Design review of the part built by this model. Coordinates are the model's own, in mm. A direction names the side the tool comes from. Coordinates: 2 decimals unless noted, no trailing zeros. Write each loop counter-clockwise with the first axis right and the second up, starting at its lowest first coordinate (ties: lowest second). Pieces come first, ordered by that corner, then holes.
Q1. Add section D-D, the plane y = 45.5. Give the boundary of the cut face in (x, z), plus the area to 3 significant figures.
Q2. To check wall thickness, follow probe 1 along X at (y, z) = (-18, 26); probe 2 along Y at (x, z) = (90.5, 26.5); probe 3 along X at (y, z) = (-51, 7). State the ranges of each line that lie inside material, in increasing order.
Q3. Add section A-A, the plane x = -84.5. Give the boundary of the cut face in (y, z).
Q4. The part is to be moulded in two halves that separate along Y. For faces 5 (the face through (-2, -61, 15)), 6 (the face through (129.035, 46.584, 15.415)), 7 (the face through (-1, -58, 0)), 8 (the face through (-129, 31, 11)), say which applies: +Y half, -Y half, draft (parallel to the pull), parting line (faces both ways), or undercut.
Q5. Machinability: for faces 1 (the face through (-116, 1, 33.4)), 2 (the face through (124.5, -17, 15)), 3 (the face through (-43.35, 36.99, 31.68)), 4 (the face through (-128.965, -43.416, 15.415)), which of the approach directions +Z, -Z, +X, -X, +Y, -Y give a long, thin tool a straight path to every point of the face, cutting with its end or side? Answer none if there is none.
Q6. Add section C-C, the plane x = -10. Give the boundary of the cut face in (y, z), plus the area to 3 significant figures.
Q7. Clearance check with flat-ended pins moving along their axes: pin 1 Ø6.5 at (x, y) = (-3, 31.5) entering from -Z; pin 2 Ø1.2 at (x, z) = (-127, 5) entering from -Y; pin 3 Ø6 at (x, z) = (22, 30.5) entering from -Y; pin 4 Ø2 at (x, y) = (99.5, -31) entering from -Z. State where each tip first meets the part, or that it passes through.
Q8. Add section B-B, the plane y = 0. Give the number of separate pieces and of enclosed holes in the cut face, plus the area to 3 significant figures.
from build123d import *

# Parameters (mm, degrees)
SKETCH1_W             = 263
SKETCH1_H             = 122
SKETCH1_W_2           = 253
SKETCH1_H_2           = 112
BOSS_EXTRUDE1_DEPTH   = 30
SKETCH1_W_3           = 249
SKETCH1_H_3           = 108
SKETCH1_W_4           = 239
SKETCH1_H_4           = 98
BOSS_EXTRUDE1_2_DEPTH = 30
SKETCH2_W             = 263
SKETCH2_H             = 122
BOSS_EXTRUDE2_DEPTH   = 5
FILLET1_R             = 1.5
SKETCH3_R             = 17.5
CUT_EXTRUDE1_DEPTH    = 12
FILLET2_R             = 3.5
FILLET3_R             = 8.5
FILLET4_R             = 5
SKETCH4_R             = 2.35
CUT_EXTRUDE2_DEPTH    = 279
SKETCH5_W             = 20
SKETCH5_H             = 35
CUT_EXTRUDE3_DEPTH    = 30
SKETCH6_W             = 7.5
SKETCH6_H             = 9
SKETCH6_W_2           = 22.5
CUT_EXTRUDE4_DEPTH    = 2.5
SKETCH7_R             = 5
CUT_EXTRUDE8_DEPTH    = 73.5
SKETCH9_R             = 3
SKETCH9_R_2           = 1.25
BOSS_EXTRUDE4_DEPTH   = 4
SKETCH10_W            = 81
SKETCH10_H            = 53
CUT_EXTRUDE9_DEPTH    = 13.6
SKETCH11_W            = 90
SKETCH11_H            = 100
CUT_EXTRUDE10_DEPTH   = 1.6
SKETCH12_W            = 70
SKETCH12_H            = 80
CUT_EXTRUDE11_DEPTH   = 11.6
FILLET5_R             = 10


with BuildPart() as part:
    # Sketch1 → Boss-Extrude1 (new body)
    with BuildSketch(Plane.XY):
        Rectangle(SKETCH1_W, SKETCH1_H)
        Rectangle(SKETCH1_W_2, SKETCH1_H_2, mode=Mode.SUBTRACT)
    extrude(amount=BOSS_EXTRUDE1_DEPTH)



with BuildPart() as body_2:
    # Sketch1 → Boss-Extrude1 2 (new body)
    with BuildSketch(Plane.XY):
        Rectangle(SKETCH1_W_3, SKETCH1_H_3)
        Rectangle(SKETCH1_W_4, SKETCH1_H_4, mode=Mode.SUBTRACT)
    extrude(amount=BOSS_EXTRUDE1_2_DEPTH)


with BuildPart() as part_1:
    add(part.part)

    add(body_2.part)  # Boss-Extrude2 merges body 2
    # Sketch2 → Boss-Extrude2 (add)
    with BuildSketch(Plane.XY.offset(30)):
        Rectangle(SKETCH2_W, SKETCH2_H)
    extrude(amount=BOSS_EXTRUDE2_DEPTH)

    # Fillet1
    fillet1_edges = [part_1.edges().sort_by_distance(p)[0] for p in [
        (-124.5, -54, 15),
        (124.5, -54, 15),
        (124.5, 54, 15),
        (-124.5, 54, 15),
    ]]
    fillet(fillet1_edges, radius=FILLET1_R)

    # Sketch3 → Cut-Extrude1 (cut)
    with BuildSketch(Plane(origin=(0, -61, 0), x_dir=(-1, 0, 0), z_dir=(0, -1, 0))):
        with Locations((105, -7.5)):
            Circle(SKETCH3_R)
        with Locations((-105, -7.5)):
            Circle(SKETCH3_R)
    extrude(amount=-CUT_EXTRUDE1_DEPTH, mode=Mode.SUBTRACT)

    # Fillet2
    fillet2_edges = [part_1.edges().sort_by_distance(p)[0] for p in [
        (126.5, 56, 15),
        (-126.5, 56, 15),
        (-126.5, -56, 15),
        (126.5, -56, 15),
    ]]
    fillet(fillet2_edges, radius=FILLET2_R)

    # Fillet3
    fillet3_edges = [part_1.edges().sort_by_distance(p)[0] for p in [
        (-131.5, -61, 17.5),
        (-131.5, 61, 17.5),
        (131.5, 61, 17.5),
        (131.5, -61, 17.5),
    ]]
    fillet(fillet3_edges, radius=FILLET3_R)

    # Fillet4
    fillet4_edges = [part_1.edges().sort_by_distance(p)[0] for p in [
        (0, -61, 35),
        (-131.5, 0, 35),
        (131.5, 0, 35),
        (0, 61, 35),
        (-129.01040764, 58.51040764, 35),
        (129.01040764, 58.51040764, 35),
        (129.01040764, -58.51040764, 35),
        (-129.01040764, -58.51040764, 35),
    ]]
    fillet(fillet4_edges, radius=FILLET4_R)

    # Sketch4 → Cut-Extrude2 (cut)
    with BuildSketch(Plane(origin=(131.5, 0, 0), x_dir=(0, 0, -1), z_dir=(1, 0, 0))):
        with Locations(Location((-17.5, -44.5, 0), (0, 0, 90))):
            Circle(SKETCH4_R)
        with Locations(Location((-17.5, 45.5, 0), (0, 0, 90))):
            Circle(SKETCH4_R)
    extrude(amount=-CUT_EXTRUDE2_DEPTH, mode=Mode.SUBTRACT)

    # Sketch5 → Cut-Extrude3 (cut)
    with BuildSketch(Plane(origin=(0, 0, 0), x_dir=(-1, 0, 0), z_dir=(0, 0, -1))):
        with Locations((114.5, 36.5)):
            Rectangle(SKETCH5_W, SKETCH5_H)
        with Locations((-114.5, 36.5)):
            Rectangle(SKETCH5_W, SKETCH5_H)
    extrude(amount=-CUT_EXTRUDE3_DEPTH, mode=Mode.SUBTRACT)

    # Sketch6 → Cut-Extrude4 (cut)
    with BuildSketch(Plane(origin=(-126.5, 0, 0), x_dir=(0, 0, -1), z_dir=(1, 0, 0))):
        with Locations((-3.75, 45.5)):
            Rectangle(SKETCH6_W, SKETCH6_H)
        with Locations((-11.25, 30.5)):
            Rectangle(SKETCH6_W_2, SKETCH6_H)
    extrude(amount=-CUT_EXTRUDE4_DEPTH, mode=Mode.SUBTRACT)

    # Sketch7 → Cut-Extrude8 (cut)
    with BuildSketch(Plane.XY.offset(30)):
        with Locations(Location((104, 20, 0), (0, 0, 180))):
            Circle(SKETCH7_R)
        with Locations(Location((104, 0, 0), (0, 0, 180))):
            Circle(SKETCH7_R)
        with Locations(Location((104, -20, 0), (0, 0, 180))):
            Circle(SKETCH7_R)
    extrude(amount=CUT_EXTRUDE8_DEPTH, mode=Mode.SUBTRACT)

    # Sketch9 → Boss-Extrude4 (add)
    # profile 1 of 4: a face of its own
    with BuildSketch(Plane(origin=(0, 0, 30), x_dir=(-1, 0, 0), z_dir=(0, 0, -1))):
        with Locations((-84.5, 32)):
            Circle(SKETCH9_R)
        with Locations((-84.5, 32)):
            Circle(SKETCH9_R_2, mode=Mode.SUBTRACT)
    # profile 2 of 4: a face of its own
    with BuildSketch(Plane(origin=(0, 0, 30), x_dir=(-1, 0, 0), z_dir=(0, 0, -1))):
        with Locations((-84.5, -32)):
            Circle(SKETCH9_R)
        with Locations((-84.5, -32)):
            Circle(SKETCH9_R_2, mode=Mode.SUBTRACT)
    # profile 3 of 4: a face of its own
    with BuildSketch(Plane(origin=(0, 0, 30), x_dir=(-1, 0, 0), z_dir=(0, 0, -1))):
        with Locations((3.5, -32)):
            Circle(SKETCH9_R)
        with Locations((3.5, -32)):
            Circle(SKETCH9_R_2, mode=Mode.SUBTRACT)
    # profile 4 of 4: a face of its own
    with BuildSketch(Plane(origin=(0, 0, 30), x_dir=(-1, 0, 0), z_dir=(0, 0, -1))):
        with Locations((3.5, 32)):
            Circle(SKETCH9_R)
        with Locations((3.5, 32)):
            Circle(SKETCH9_R_2, mode=Mode.SUBTRACT)
    extrude(amount=BOSS_EXTRUDE4_DEPTH)

    # Sketch10 → Cut-Extrude9 (cut)
    with BuildSketch(Plane(origin=(0, 0, 30), x_dir=(-1, 0, 0), z_dir=(0, 0, -1))):
        with Locations((-40.5, 0)):
            Rectangle(SKETCH10_W, SKETCH10_H)
    extrude(amount=-CUT_EXTRUDE9_DEPTH, mode=Mode.SUBTRACT)

    # Sketch11 → Cut-Extrude10 (cut)
    with BuildSketch(Plane.XY.offset(35)):
        with Locations((-75.5, 0)):
            Rectangle(SKETCH11_W, SKETCH11_H)
    extrude(amount=-CUT_EXTRUDE10_DEPTH, mode=Mode.SUBTRACT)

    # Sketch12 → Cut-Extrude11 (cut)
    with BuildSketch(Plane.XY.offset(33.4)):
        with Locations((-75.5, 0)):
            Rectangle(SKETCH12_W, SKETCH12_H)
    extrude(amount=-CUT_EXTRUDE11_DEPTH, mode=Mode.SUBTRACT)

    # Fillet5
    fillet5_edges = [part_1.edges().sort_by_distance(p)[0] for p in [
        (-30.5, 50, 34.2),
        (-30.5, -50, 34.2),
        (-120.5, -50, 34.2),
        (-120.5, 50, 34.2),
        (-110.5, -40, 31.7),
        (-110.5, 40, 31.7),
        (-40.5, 40, 31.7),
        (-40.5, -40, 31.7),
    ]]
    fillet(fillet5_edges, radius=FILLET5_R)


solid = part_1.part
Here are the results:
1. outline: (-131.5, 0) - (-129, 0) - (-129, 7.5) - (-126.5, 7.5) - (-126.5, 15.15) - (-131.5, 15.15) - close; (-131.5, 19.85) - (-126.5, 19.85) - (-126.5, 30) - (126.5, 30) - (126.5, 19.85) - (131.5, 19.85) - (131.5, 30) arc R5 ccw to (126.5, 35) - (-32.15, 35) - (-32.15, 33.4) - (-118.85, 33.4) - (-118.85, 35) - (-126.5, 35) arc R5 ccw to (-131.5, 30) - close; (126.5, 0) - (131.5, 0) - (131.5, 15.15) - (126.5, 15.15) - close
1. area: 1,400 mm2
2. probe 1: x = -131.5 to -126.5, -124.5 to -119.5, 119.5 to 124.5, 126.5 to 131.5
2. probe 2: y = -61 to -56, -54 to -49, 49 to 54, 56 to 61
2. probe 3: x = -131.5 to -126.5, -124.5 to -122.49, -87.51 to 87.51, 122.49 to 124.5, 126.5 to 131.5
3. outline: (-61, 0) - (-56, 0) - (-56, 30) - (-54, 30) - (-54, 0) - (-49, 0) - (-49, 30) - (-40, 30) - (-40, 33.4) - (-50, 33.4) - (-50, 35) - (-56, 35) arc R5 ccw to (-61, 30) - close; (40, 30) - (49, 30) - (49, 0) - (54, 0) - (54, 30) - (56, 30) - (56, 0) - (61, 0) - (61, 30) arc R5 ccw to (56, 35) - (50, 35) - (50, 33.4) - (40, 33.4) - close
4. face 5: -Y half
4. face 6: undercut
4. face 7: draft
4. face 8: undercut
5. face 1: +Z
5. face 2: -Z
5. face 3: +Z, -Z
5. face 4: +X, -X
6. outline: (-61, 0) - (-56, 0) - (-56, 30) - (-54, 30) - (-54, 0) - (-49, 0) - (-49, 30) - (49, 30) - (49, 0) - (54, 0) - (54, 30) - (56, 30) - (56, 0) - (61, 0) - (61, 30) arc R5 ccw to (56, 35) - (-56, 35) arc R5 ccw to (-61, 30) - close
6. area: 1,200 mm2
7. pin 1: stops at z = 26
7. pin 2: stops at y = -60.29
7. pin 3: stops at y = -61
7. pin 4: stops at z = 30
8. separate pieces: 4
8. enclosed holes: 0
8. area: 1,070 mm2
